Source: CAD feature listing. Evaluate the final solid. Frame: model axes, mm. A direction names the side the tool comes from. Coordinates: 2 decimals unless noted, no trailing zeros. Order: outer loops, then holes, each group sorted by start corner. A loop starts at its lowest first (then second) coordinate and runs counter-clockwise, first axis right, second up.
Autodesk Inventor part; units mm, degrees
ref_plane "Work Plane1" through (-76.2, 50.8, 9.525) normal (0, 0, 1) x (1, 0, 0)
ref_plane "YZ Plane" through (0, 0, 0) normal (1, 0, 0) x (0, 1, 0)
ref_plane "XZ Plane" through (0, 0, 0) normal (0, 1, 0) x (-1, 0, 0)
sketch "Sketch1" plane through (0, 0, 0) normal (0, 0, 1) x (1, 0, 0)
  line L0 (-76.2, -50.8) -> (76.2, -50.8)
  line L1 (76.2, -50.8) -> (76.2, 50.8)
  line L2 (76.2, 50.8) -> (-76.2, 50.8)
  line L3 (-76.2, 50.8) -> (-76.2, -50.8)
  line L4 (-76.2, -50.8) -> (76.2, 50.8) construction
  line L5 (76.2, -50.8) -> (-76.2, 50.8) construction
  point P0 (0, 0)
  dimension "d0" = 152.4
  dimension "d1" = 101.6
extrude "Extrusion1" add sketch "Sketch1" along normal mid plane 19.05
sketch "Sketch3" plane through (0, 0, 9.525) normal (0, 0, 1) x (1, 0, 0)
  line L0 (-76.2, -12.7) -> (76.2, -12.7)
  line L1 (76.2, -12.7) -> (76.2, 12.7)
  line L2 (76.2, 12.7) -> (-76.2, 12.7)
  line L3 (-76.2, 12.7) -> (-76.2, -12.7)
  line L4 (-76.2, -12.7) -> (76.2, 12.7) construction
  line L5 (76.2, -12.7) -> (-76.2, 12.7) construction
  point P0 (0, 0)
  dimension "d7" = 25.4
  dimension "d19" = 152.4
extrude "Extrusion3" cut sketch "Sketch3" against normal blind 12.7
ref_plane "Work Plane1" through (-76.2, 50.8, 9.525) normal (0, 0, 1) x (1, 0, 0)
sketch "Sketch8" plane through (0, 0, 9.525) normal (0, 0, 1) x (1, 0, 0)
  line L0 (-76.2, -12.7) -> (-76.2, 12.7)
  line L1 (-76.2, 0) -> (38.1, 0)
  line L2 (38.1, 0) -> (38.1, 38.1)
  line L3 (38.1, 38.1) -> (-76.2, 38.1)
  line L4 (-76.2, 38.1) -> (-76.2, 0)
  line L5 (38.1, 0) -> (38.1, -38.1)
  line L6 (38.1, -38.1) -> (-76.2, -38.1)
  line L7 (-76.2, -38.1) -> (-76.2, 0)
  point P0 (0, 0)
  dimension "d51" = 114.3
  dimension "d52" = 38.1
extrude "Extrusion6" cut sketch "Sketch8" against normal blind 7.366
sketch "Sketch9" plane through (0, 0, 9.525) normal (0, 0, 1) x (1, 0, 0)
  line L0 (-76.2, 50.8) -> (-76.2, 38.1) construction
  line L1 (-76.2, 44.45) -> (76.2, 44.45) construction
  line L2 (76.2, 50.8) -> (76.2, -50.8) construction
  line L3 (-76.2, 44.45) -> (-76.2, -44.4609) construction
  point P0 (0, 0)
  point P1 (-50.8, 44.45)
  point P2 (-25.4, 44.45)
  point P3 (0, 44.45)
  point P4 (25.4, 44.45)
  point P5 (50.8, 44.45)
  point P6 (-50.8, -44.45)
  point P7 (-25.4, -44.45)
  point P8 (0, -44.45)
  point P9 (25.4, -44.45)
  point P10 (50.8, -44.45)
  point P11 (-50.8, -133.35)
  point P12 (-25.4, -133.35)
  point P13 (0, -133.35)
  point P14 (25.4, -133.35)
  point P15 (50.8, -133.35)
  point P16 (-50.8, -222.25)
  point P17 (-25.4, -222.25)
  point P18 (0, -222.25)
  point P19 (25.4, -222.25)
  point P20 (50.8, -222.25)
  dimension "d55" = 25.4
  dimension "d58" = 25.4
  dimension "d61" = 88.9
hole "Hole2" at (-50.8, 44.45, 9.525) at (-25.4, 44.45, 9.525) at (0, 44.45, 9.525) at (25.4, 44.45, 9.525) at (50.8, 44.45, 9.525) at (-50.8, -44.45, 9.525) at (-25.4, -44.45, 9.525) at (0, -44.45, 9.525) at (25.4, -44.45, 9.525) at (50.8, -44.45, 9.525) at (-50.8, -133.35, 9.525) at (-25.4, -133.35, 9.525) at (0, -133.35, 9.525) at (25.4, -133.35, 9.525) at (50.8, -133.35, 9.525) at (-50.8, -222.25, 9.525) at (-25.4, -222.25, 9.525) at (0, -222.25, 9.525) at (25.4, -222.25, 9.525) at (50.8, -222.25, 9.525) direction (0, 0, -1) diameter 5.1054 end through all
properties part number "pistonHousing" material "PET Plastic"
1. Section query A-A on z = 6.75. Count the separate pieces of the cut face and the enclosed holes in it, plus the area to 3 significant figures.
Findings:
separate pieces: 2
enclosed holes: 10
area: 5,600 mm2
2. Ray query, line 1 (X direction, y = 44.45, z = 1.75); line 2 (Y direction, x = 25.4, z = -5.25); line 3 (Y direction, x = 44.5, z = 7). Return the intervals inside material, ascending.
Findings:
line 1: x = -76.2 to -53.35, -48.25 to -27.95, -22.85 to -2.55, 2.55 to 22.85, 27.95 to 48.25, 53.35 to 76.2
line 2: y = -50.8 to -47, -41.9 to 41.9, 47 to 50.8
line 3: y = -50.8 to -12.7, 12.7 to 50.8
3. Section query B-B on y = 44.45. Return loops of the section in (x, z) (3 decimals).
Findings:
outline: (-76.2, -9.525) - (-53.353, -9.525) - (-53.353, 9.525) - (-76.2, 9.525) - close; (-48.247, -9.525) - (-27.953, -9.525) - (-27.953, 9.525) - (-48.247, 9.525) - close; (-22.847, -9.525) - (-2.553, -9.525) - (-2.553, 9.525) - (-22.847, 9.525) - close; (2.553, -9.525) - (22.847, -9.525) - (22.847, 9.525) - (2.553, 9.525) - close; (27.953, -9.525) - (48.247, -9.525) - (48.247, 9.525) - (27.953, 9.525) - close; (53.353, -9.525) - (76.2, -9.525) - (76.2, 9.525) - (53.353, 9.525) - close
4. Pin query (flat end, axial travel): P1, Ø20.5, axis at x = -8.5, y = 1, coming from the +Z side (3 decimals); P2, Ø6, axis at x = -25.4, y = -44.45, coming from the +Z side (3 decimals); P3, Ø12.5, axis at x = -6, y = 28, coming from the +Z side. Return the tip coordinate at first contact, or that it passes through.
Findings:
P1: stops at z = -3.175
P2: stops at z = 9.525
P3: stops at z = 2.16
5. Draft query along Y for faces 1 (the face through (16, 40, 9.525)), 2 (the face through (-18, -38.1, 6)). Return one class per face: released by +Y, released by -Y, zero draft, split by the parting line, or undercut.
Findings:
face 1: zero draft
face 2: undercut
6. Access query for faces 3 (the face through (38.1, 26, 6)), 4 (the face through (18, 12.7, 0)), 5 (the face through (-0.767, 42.015, -0.133)). Directions: +Z, -Z, +X, -X, +Y, -Y. A direction counts if a zero-diameter tool reaches every point of the face in a straight line with its end or side. Return the directions, or none.
Findings:
face 3: +Z, -X
face 4: +Z, +X, -X
face 5: +Z, -Z
7. Section query C-C on x = 50.8. Return loops of the section in (y, z) (3 decimals).
Findings:
outline: (-50.8, -9.525) - (-47.003, -9.525) - (-47.003, 9.525) - (-50.8, 9.525) - close; (-41.897, -9.525) - (41.897, -9.525) - (41.897, 9.525) - (12.7, 9.525) - (12.7, -3.175) - (-12.7, -3.175) - (-12.7, 9.525) - (-41.897, 9.525) - close; (47.003, -9.525) - (50.8, -9.525) - (50.8, 9.525) - (47.003, 9.525) - close
8. Section query D-D on x = 13. Return loops of the section in (y, z) (3 decimals), plus the area to 3 significant figures.
Findings:
outline: (-50.8, -9.525) - (50.8, -9.525) - (50.8, 9.525) - (38.1, 9.525) - (38.1, 2.159) - (12.7, 2.159) - (12.7, -3.175) - (-12.7, -3.175) - (-12.7, 2.159) - (-38.1, 2.159) - (-38.1, 9.525) - (-50.8, 9.525) - close
area: 1,240 mm2
